```python
from build123d import *

# Parameters (mm, degrees)
F1_DEPTH = 60


with BuildPart() as f1:
    # F0 (on Front) → F1 (new body)
    with BuildSketch(Plane.XZ):
        Polygon((0, 25), (0, 0), (20, 0), (100, 0), (120, 0), (120, 18.918289), (38.999476, 46.372868), align=None)
        with BuildLine():
            ThreePointArc((21.075, 10), (20.76014, 9.23986), (20, 8.925))
            ThreePointArc((20, 8.925), (19.23986, 10.76014), (21.075, 10))
        make_face(mode=Mode.SUBTRACT)
        with BuildLine():
            ThreePointArc((101.075, 10), (100.76014, 9.23986), (100, 8.925))
            ThreePointArc((100, 8.925), (99.23986, 10.76014), (101.075, 10))
        make_face(mode=Mode.SUBTRACT)
    extrude(amount=F1_DEPTH)


solid = f1.part
```
Source: CAD feature listing. Evaluate the final solid. Frame: model axes, mm. Round coordinates to 2 decimals unless told otherwise and drop trailing zeros. Loops run counter-clockwise (first coordinate to the right, second up) from the corner with the lowest first, then second, coordinate; pieces in that order, holes last. Notation, with made-up numbers: M 44,-0.5 L 73,-0.5 A28 cw 73,33.5 Z; hole C -0.5,28 d4. An arc over 180 degrees is marked long. Use a Markdown table: item, result. Add a question column.
1. Ray query, line 1 along X through (y, z) = (-45.5, 10) (3 decimals); line 2 along X through (y, z) = (-44.5, 9.5); line 3 along Z through (x, y) = (20, -14) (3 decimals). Return the intervals inside material, ascending. Write a range as [from, to].
2. Cut plane C-C, the plane x = 44. Output: boundary loops of the cut face in (y, z).
3. Cut plane A-A, the plane y = -33.5. Output: boundary loops of the cut face in (x, z) (3 decimals), and give its area (3 significant figures).
4. Cut plane B-B, the plane z = 41.5. Output: boundary loops of the cut face in (x, y), and give its area (3 significant figures).
5. Contact query for flat-ended pins moving along their axis: pin 1 (3 mm diameter, centred on x = 94, y = -37.5, fed in from +Z); pin 2 (1.5 mm diameter, centred on x = 93, y = -32.5, fed in from +Z); pin 3 (2 mm diameter, centred on y = -49.5, z = 27.5, fed in from -X); pin 4 (1.9 mm diameter, centred on x = 100, z = 10, fed in from +Y). Output: stop coordinate, or through.
Solution:
| question | item | result |
|---|---|---|
| 1 | line 1 | x = [0, 18.925], [21.075, 98.925], [101.075, 120] |
| 1 | line 2 | x = [0, 19.05], [20.95, 99.05], [100.95, 120] |
| 1 | line 3 | z = [0, 8.925], [11.075, 35.961] |
| 2 | outline | M -60,0 L 0,0 L 0,44.68 L -60,44.68 Z |
| 3 | outline | M 0,0 L 120,0 L 120,18.918 L 38.999,46.373 L 0,25 Z; hole C 20,10 d2.15; hole C 100,10 d2.15 |
| 3 | area | 4,030 mm2 |
| 4 | outline | M 30.11,-60 L 53.38,-60 L 53.38,0 L 30.11,0 Z |
| 4 | area | 1,400 mm2 |
| 5 | pin 1 | stops at z = 28.24 |
| 5 | pin 2 | stops at z = 28.32 |
| 5 | pin 3 | stops at x = 2.74 |
| 5 | pin 4 | passes through |
